Could you check a few things on this model? Use its own coordinates, in mm. Give positions to 0.01 mm unless a question says otherwise; leave off trailing zeros. Order: outer loops, then holes, each group sorted by start corner. A loop starts at its lowest first (then second) coordinate and runs counter-clockwise, first axis right, second up.
from build123d import *

# Parameters (mm, degrees)
SKETCH1_R           = 95.25
SKETCH1_R_2         = 66.675
MAIN_ROTOR_DEPTH    = 4.7625
SKETCH2_R           = 2.38125
CUT_SLOTS_DEPTH     = 135.788005424
BOSS_EXTRUDE2_START = -4.7625
BOSS_EXTRUDE2_DEPTH = 4.7625
SKETCH4_R           = 1.27
CUT_EXTRUDE2_DEPTH  = 135.788005424
FE12_CUT_OUT_DEPTH  = 4.7625
CIRPATTERN1_COUNT   = 6
SKETCH7_R           = 46.99
CLEANUP_CUT_DEPTH   = 135.788005424


with BuildPart() as part:
    # Sketch1 → Main Rotor (new body)
    with BuildSketch(Plane(origin=(0, 0, 0), x_dir=(0, 0, -1), z_dir=(1, 0, 0))):
        with Locations(Location((0, 0, 0), (0, 0, 180))):
            Circle(SKETCH1_R)
        with Locations(Location((0, 0, 0), (0, 0, 180))):
            Circle(SKETCH1_R_2, mode=Mode.SUBTRACT)
    extrude(amount=MAIN_ROTOR_DEPTH)

    # Sketch2 → Cut Slots (cut, through all)
    with BuildSketch(Plane(origin=(4.7625, 0, 0), x_dir=(0, 0, -1), z_dir=(1, 0, 0))):
        with Locations((-80.045174165, 14.114123881)):
            Circle(SKETCH2_R)
        with Locations((-82.345264359, 29.97122516)):
            Circle(SKETCH2_R)
        with Locations((-70.411168075, 25.627569339)):
            Circle(SKETCH2_R)
        with Locations((-70.39054482, 40.64)):
            Circle(SKETCH2_R)
        with Locations((-67.128474551, 56.327478237)):
            Circle(SKETCH2_R)
        with Locations((-57.399710123, 48.164075594)):
            Circle(SKETCH2_R)
        with Locations((-52.245776915, 62.264092337)):
            Circle(SKETCH2_R)
        with Locations((-87.63, 0)):
            Circle(SKETCH2_R)
        with Locations((-43.815, 75.889806134)):
            Circle(SKETCH2_R)
        with Locations((-37.465, 64.891283506)):
            Circle(SKETCH2_R)
        with Locations((-74.93, 0)):
            Circle(SKETCH2_R)
        with Locations((-27.79939725, 76.378216217)):
            Circle(SKETCH2_R)
        with Locations((-15.216789809, 86.298703396)):
            Circle(SKETCH2_R)
        with Locations((-13.011457953, 73.791644933)):
            Circle(SKETCH2_R)
        with Locations((0, 81.28)):
            Circle(SKETCH2_R)
        with Locations((15.216789809, 86.298703396)):
            Circle(SKETCH2_R)
        with Locations((13.011457953, 73.791644933)):
            Circle(SKETCH2_R)
        with Locations((27.79939725, 76.378216217)):
            Circle(SKETCH2_R)
        with Locations((43.815, 75.889806134)):
            Circle(SKETCH2_R)
        with Locations((37.465, 64.891283506)):
            Circle(SKETCH2_R)
        with Locations((52.245776915, 62.264092337)):
            Circle(SKETCH2_R)
        with Locations((67.128474551, 56.327478237)):
            Circle(SKETCH2_R)
        with Locations((57.399710123, 48.164075594)):
            Circle(SKETCH2_R)
        with Locations((70.39054482, 40.64)):
            Circle(SKETCH2_R)
        with Locations((82.345264359, 29.97122516)):
            Circle(SKETCH2_R)
        with Locations((70.411168075, 25.627569339)):
            Circle(SKETCH2_R)
        with Locations((80.045174165, 14.114123881)):
            Circle(SKETCH2_R)
        with Locations((87.63, 0)):
            Circle(SKETCH2_R)
        with Locations((74.93, 0)):
            Circle(SKETCH2_R)
        with Locations((80.045174165, -14.114123881)):
            Circle(SKETCH2_R)
        with Locations((82.345264359, -29.97122516)):
            Circle(SKETCH2_R)
        with Locations((70.411168075, -25.627569339)):
            Circle(SKETCH2_R)
        with Locations((70.39054482, -40.64)):
            Circle(SKETCH2_R)
        with Locations((67.128474551, -56.327478237)):
            Circle(SKETCH2_R)
        with Locations((57.399710123, -48.164075594)):
            Circle(SKETCH2_R)
        with Locations((52.245776915, -62.264092337)):
            Circle(SKETCH2_R)
        with Locations((43.815, -75.889806134)):
            Circle(SKETCH2_R)
        with Locations((37.465, -64.891283506)):
            Circle(SKETCH2_R)
        with Locations((27.79939725, -76.378216217)):
            Circle(SKETCH2_R)
        with Locations((15.216789809, -86.298703396)):
            Circle(SKETCH2_R)
        with Locations((13.011457953, -73.791644933)):
            Circle(SKETCH2_R)
        with Locations((0, -81.28)):
            Circle(SKETCH2_R)
        with Locations((-15.216789809, -86.298703396)):
            Circle(SKETCH2_R)
        with Locations((-13.011457953, -73.791644933)):
            Circle(SKETCH2_R)
        with Locations((-27.79939725, -76.378216217)):
            Circle(SKETCH2_R)
        with Locations((-43.815, -75.889806134)):
            Circle(SKETCH2_R)
        with Locations((-37.465, -64.891283506)):
            Circle(SKETCH2_R)
        with Locations((-52.245776915, -62.264092337)):
            Circle(SKETCH2_R)
        with Locations((-67.128474551, -56.327478237)):
            Circle(SKETCH2_R)
        with Locations((-57.399710123, -48.164075594)):
            Circle(SKETCH2_R)
        with Locations((-70.39054482, -40.64)):
            Circle(SKETCH2_R)
        with Locations((-82.345264359, -29.97122516)):
            Circle(SKETCH2_R)
        with Locations((-70.411168075, -25.627569339)):
            Circle(SKETCH2_R)
        with Locations((-80.045174165, -14.114123881)):
            Circle(SKETCH2_R)
    extrude(amount=-CUT_SLOTS_DEPTH, mode=Mode.SUBTRACT)

    # Sketch3 → Boss-Extrude2 (add)
    with BuildSketch(Plane(origin=(4.7625, 0, 0), x_dir=(0, 0, -1), z_dir=(1, 0, 0)).offset(BOSS_EXTRUDE2_START)):
        with BuildLine():
            ThreePointArc((15.226370254, -60.56863172), (10.49630902, -58.039692226), (8.604258147, -53.0208121))
            ThreePointArc((8.604258147, -53.0208121), (11.546477683, -42.011879168), (19.60245, -33.952439353))
            ThreePointArc((19.60245, -33.952439353), (30.610115778, -31.005482581), (41.615241134, -33.961912186))
            ThreePointArc((41.615241134, -33.961912186), (45.015693386, -38.109916371), (44.840788615, -43.470739307))
            ThreePointArc((44.840788615, -43.470739307), (40.527102575, -50.964468228), (34.431304095, -57.096768064))
            ThreePointArc((34.431304095, -57.096768064), (57.742243797, -33.3375), (66.662903665, -1.27))
            ThreePointArc((66.662903665, -1.27), (64.400075463, -9.615266258), (60.067158869, -17.097892412))
            ThreePointArc((60.067158869, -17.097892412), (55.512002406, -19.929775856), (50.219499281, -19.058899914))
            ThreePointArc((50.219499281, -19.058899914), (42.156593461, -11.006396586), (39.2049, 0))
            ThreePointArc((39.2049, 0), (42.156593461, 11.006396586), (50.219499281, 19.058899914))
            ThreePointArc((50.219499281, 19.058899914), (55.512002406, 19.929775856), (60.067158869, 17.097892412))
            ThreePointArc((60.067158869, 17.097892412), (64.400075463, 9.615266258), (66.662903665, 1.27))
            ThreePointArc((66.662903665, 1.27), (57.742243797, 33.3375), (34.431304095, 57.096768064))
            ThreePointArc((34.431304095, 57.096768064), (40.527102575, 50.964468228), (44.840788615, 43.470739307))
            ThreePointArc((44.840788615, 43.470739307), (45.015693386, 38.109916371), (41.615241134, 33.961912186))
            ThreePointArc((41.615241134, 33.961912186), (30.610115778, 31.005482581), (19.60245, 33.952439353))
            ThreePointArc((19.60245, 33.952439353), (11.546477683, 42.011879168), (8.604258147, 53.0208121))
            ThreePointArc((8.604258147, 53.0208121), (10.49630902, 58.039692226), (15.226370254, 60.56863172))
            ThreePointArc((15.226370254, 60.56863172), (23.872972888, 60.579734486), (32.23159957, 58.366768064))
            ThreePointArc((32.23159957, 58.366768064), (0, 66.675), (-32.23159957, 58.366768064))
            ThreePointArc((-32.23159957, 58.366768064), (-23.872972888, 60.579734486), (-15.226370254, 60.56863172))
            ThreePointArc((-15.226370254, 60.56863172), (-10.49630902, 58.039692226), (-8.604258147, 53.0208121))
            ThreePointArc((-8.604258147, 53.0208121), (-11.546477683, 42.011879168), (-19.60245, 33.952439353))
            ThreePointArc((-19.60245, 33.952439353), (-30.610115778, 31.005482581), (-41.615241134, 33.961912186))
            ThreePointArc((-41.615241134, 33.961912186), (-45.015693386, 38.109916371), (-44.840788615, 43.470739307))
            ThreePointArc((-44.840788615, 43.470739307), (-40.527102575, 50.964468228), (-34.431304095, 57.096768064))
            ThreePointArc((-34.431304095, 57.096768064), (-57.742243797, 33.3375), (-66.662903665, 1.27))
            ThreePointArc((-66.662903665, 1.27), (-64.400075463, 9.615266258), (-60.067158869, 17.097892412))
            ThreePointArc((-60.067158869, 17.097892412), (-55.512002406, 19.929775856), (-50.219499281, 19.058899914))
            ThreePointArc((-50.219499281, 19.058899914), (-42.156593461, 11.006396586), (-39.2049, 0))
            ThreePointArc((-39.2049, 0), (-42.156593461, -11.006396586), (-50.219499281, -19.058899914))
            ThreePointArc((-50.219499281, -19.058899914), (-55.512002406, -19.929775856), (-60.067158869, -17.097892412))
            ThreePointArc((-60.067158869, -17.097892412), (-64.400075463, -9.615266258), (-66.662903665, -1.27))
            ThreePointArc((-66.662903665, -1.27), (-57.742243797, -33.3375), (-34.431304095, -57.096768064))
            ThreePointArc((-34.431304095, -57.096768064), (-40.527102575, -50.964468228), (-44.840788615, -43.470739307))
            ThreePointArc((-44.840788615, -43.470739307), (-45.015693386, -38.109916371), (-41.615241134, -33.961912186))
            ThreePointArc((-41.615241134, -33.961912186), (-30.610115778, -31.005482581), (-19.60245, -33.952439353))
            ThreePointArc((-19.60245, -33.952439353), (-11.546477683, -42.011879168), (-8.604258147, -53.0208121))
            ThreePointArc((-8.604258147, -53.0208121), (-10.49630902, -58.039692226), (-15.226370254, -60.56863172))
            ThreePointArc((-15.226370254, -60.56863172), (-23.872972888, -60.579734486), (-32.23159957, -58.366768064))
            ThreePointArc((-32.23159957, -58.366768064), (0, -66.675), (32.23159957, -58.366768064))
            ThreePointArc((32.23159957, -58.366768064), (23.872972888, -60.579734486), (15.226370254, -60.56863172))
        make_face()
        with BuildLine():
            Line((-16.8148, 11.541116411), (-1.5875, 20.332602165))
            ThreePointArc((-1.5875, 20.332602165), (0, 21.920102165), (1.5875, 20.332602165))
            Line((1.5875, 20.332602165), (16.8148, 11.541116411))
            ThreePointArc((16.8148, 11.541116411), (18.4023, 11.541116411), (19.19605, 10.166301083))
            ThreePointArc((19.19605, 10.166301083), (18.983365329, 9.372551083), (18.4023, 8.791485754))
            Line((18.4023, 8.791485754), (18.4023, -8.791485754))
            ThreePointArc((18.4023, -8.791485754), (18.983365329, -9.372551083), (19.19605, -10.166301083))
            ThreePointArc((19.19605, -10.166301083), (18.4023, -11.541116411), (16.8148, -11.541116411))
            Line((16.8148, -11.541116411), (1.5875, -20.332602165))
            ThreePointArc((1.5875, -20.332602165), (0, -21.920102165), (-1.5875, -20.332602165))
            Line((-1.5875, -20.332602165), (-16.8148, -11.541116411))
            ThreePointArc((-16.8148, -11.541116411), (-18.983365329, -10.960051083), (-18.4023, -8.791485754))
            Line((-18.4023, -8.791485754), (-18.4023, 8.791485754))
            ThreePointArc((-18.4023, 8.791485754), (-18.983365329, 10.960051083), (-16.8148, 11.541116411))
        make_face(mode=Mode.SUBTRACT)
    extrude(amount=BOSS_EXTRUDE2_DEPTH)

    # Sketch4 → Cut-Extrude2 (cut, through all)
    with BuildSketch(Plane.ZY):
        with Locations((0, 45.212)):
            Circle(SKETCH4_R)
        with Locations((39.154740556, 22.606)):
            Circle(SKETCH4_R)
        with Locations((39.154740556, -22.606)):
            Circle(SKETCH4_R)
        with Locations((0, -45.212)):
            Circle(SKETCH4_R)
        with Locations((-39.154740556, -22.606)):
            Circle(SKETCH4_R)
        with Locations((-39.154740556, 22.606)):
            Circle(SKETCH4_R)
    extrude(amount=-CUT_EXTRUDE2_DEPTH, mode=Mode.SUBTRACT)

    # Sketch6 → FE12 Cut OUt (cut)
    with BuildSketch(Plane(origin=(4.7625, 0, 0), x_dir=(0, 0, -1), z_dir=(1, 0, 0))):
        with BuildLine():
            Line((-18.4023, 60.5917), (-5.950469261, 60.5917))
            ThreePointArc((-5.950469261, 60.5917), (0, 66.367025), (5.950469261, 60.5917))
            Line((5.950469261, 60.5917), (18.4023, 60.5917))
            Line((18.4023, 60.5917), (18.4023, 35.1917))
            Line((18.4023, 35.1917), (-18.4023, 35.1917))
            Line((-18.4023, 35.1917), (-18.4023, 60.5917))
        make_face()
    fe12_cut_out = extrude(amount=-FE12_CUT_OUT_DEPTH, mode=Mode.SUBTRACT)

    # CirPattern1: FE12 Cut OUt ×6 about axis
    cirpattern1_axis = Axis((0, 0, 0), (1, 0, 0))
    for i in range(1, CIRPATTERN1_COUNT):
        add(fe12_cut_out.rotate(cirpattern1_axis, i * 360 / CIRPATTERN1_COUNT), mode=Mode.SUBTRACT)

    # Sketch7 → Cleanup Cut (cut, through all)
    with BuildSketch(Plane(origin=(4.7625, 0, 0), x_dir=(0, 0, -1), z_dir=(1, 0, 0))):
        Circle(SKETCH7_R)
    extrude(amount=-CLEANUP_CUT_DEPTH, mode=Mode.SUBTRACT)


solid = part.part
Item 1: For pin 1 (6 mm diameter, centred on y = -25.63, z = 70.41, fed in from -X); pin 2 (4 mm diameter, centred on y = 75.89, z = -43.82, fed in from +X); pin 3 (2 mm diameter, centred on x = 3, z = -19.5, fed in from -Y); pin 4 (2.5 mm diameter, centred on x = 3.5, z = 12.5, fed in from -Y), each with a flat end and sliding along its axis, tell me the tip position at first contact or that it passes through.
Findings:
pin 1: stops at x = 0
pin 2: passes through
pin 3: stops at y = -93.44
pin 4: stops at y = -94.58
Item 2: We'd pull the mould along Z, two halves only. Please class faces 1 (the flat face through (2.415, 21.106, -57.78)), 2 (the flat face through (4.762, 20, 62)), 3 (the cylindrical face through (2.348, 92.985, -20.648)): +Z half, -Z half, draft (parallel to the pull), parting line (faces both ways), or undercut.
Findings:
face 1: undercut
face 2: draft
face 3: parting line
Item 3: Imagine slicing it at D-D on x = 3.95. Give the number of separate pieces and of enclosed holes in the cut face, then the cut area to 3 significant figures.
Findings:
separate pieces: 1
enclosed holes: 55
area: 14,600 mm2
Item 4: Imagine slicing it at C-C on y = -40.64. List the corners of the cut face in (x, z) for me, then the cut area to 3 significant figures.
Findings:
outline: (0, -86.14) - (4.76, -86.14) - (4.76, -72.77) - (0, -72.77) - close; (0, -68.01) - (4.76, -68.01) - (4.76, -46.5) - (0, -46.5) - close; (0, 46.5) - (4.76, 46.5) - (4.76, 68.01) - (0, 68.01) - close; (0, 72.77) - (4.76, 72.77) - (4.76, 86.14) - (0, 86.14) - close
area: 332 mm2
Item 5: Please list where these lines run through material, in increasing order: line 1 along Y through (x, z) = (3.05, 0); line 2 along Y through (x, z) = (1.15, -51); line 3 along Y through (x, z) = (4.3, -75).
Findings:
line 1: y = -95.25 to -83.66, -78.9 to -66.37, 66.37 to 78.9, 83.66 to 95.25
line 2: y = -80.45 to -64.29, -60.23 to -36.01, 36.01 to 60.23, 64.29 to 80.45
line 3: y = -58.72 to -2.38, 2.38 to 58.72
Item 6: Imagine slicing it at B-B on y = 81.28. List the corners of the cut face in (x, z) for me, then the cut area to 3 significant figures.
Findings:
outline: (0, -49.66) - (4.76, -49.66) - (4.76, -2.38) - (0, -2.38) - close; (0, 2.38) - (4.76, 2.38) - (4.76, 49.66) - (0, 49.66) - close
area: 450 mm2
Item 7: Imagine slicing it at A-A on z = -28. List the corners of the cut face in (x, y) for me, then the cut area to 3 significant figures.
Findings:
outline: (0, -91.04) - (4.76, -91.04) - (4.76, -78.75) - (0, -78.75) - close; (0, -74.01) - (4.76, -74.01) - (4.76, -59.78) - (0, -59.78) - close; (0, 59.78) - (4.76, 59.78) - (4.76, 74.01) - (0, 74.01) - close; (0, 78.75) - (4.76, 78.75) - (4.76, 91.04) - (0, 91.04) - close
area: 253 mm2
